from build123d import *

# Parameters (mm, degrees)
SKETCH1_W           = 14.0208
SKETCH1_H           = 7.62
BOSS_EXTRUDE1_DEPTH = 1.3081
SKETCH2_W           = 0.762
SKETCH2_H           = 0.762
CUT_EXTRUDE1_DEPTH  = 6.35
CHAMFER1_SIZE       = 0.508
SKETCH3_W           = 1.778
SKETCH3_H           = 1.778
CUT_EXTRUDE2_DEPTH  = 0.254
SKETCH4_R           = 0.762
CUT_EXTRUDE3_DEPTH  = 5.08
SKETCH5_W           = 5.0038
SKETCH5_H           = 0.6604
CUT_EXTRUDE4_DEPTH  = 8.62
SKETCH6_W           = 1.524
SKETCH6_H           = 0.381
SKETCH6_H_2         = 0.762
SKETCH6_H_3         = 1.524
CUT_EXTRUDE5_DEPTH  = 0.254
SKETCH7_W           = 1.524
SKETCH7_H           = 0.254
BOSS_EXTRUDE2_DEPTH = 3.4798
SKETCH8_W           = 0.762
SKETCH8_H           = 0.762
BOSS_EXTRUDE3_DEPTH = 12.7
CHAMFER2_SIZE       = 0.254


with BuildPart() as part:
    # Sketch1 → Boss-Extrude1 (new body, symmetric)
    with BuildSketch(Plane(origin=(0, 0, 0), x_dir=(1, 0, 0), z_dir=(0, 1, 0))):
        Rectangle(SKETCH1_W, SKETCH1_H)
    extrude(amount=BOSS_EXTRUDE1_DEPTH, both=True)

    # Sketch2 → Cut-Extrude1 (cut)
    with BuildSketch(Plane(origin=(7.0104, 0, 0), x_dir=(0, 0, -1), z_dir=(1, 0, 0))):
        Rectangle(SKETCH2_W, SKETCH2_H)
        with Locations((-2.54, 0)):
            Rectangle(SKETCH2_W, SKETCH2_H)
        with Locations((2.54, 0)):
            Rectangle(SKETCH2_W, SKETCH2_H)
    extrude(amount=-CUT_EXTRUDE1_DEPTH, mode=Mode.SUBTRACT)

    # Chamfer1
    chamfer1_edges = [part.edges().sort_by_distance(p)[0] for p in [
        (7.0104, -0.381, 2.54),
        (7.0104, 0, 2.159),
        (7.0104, 0.381, 2.54),
        (7.0104, 0, 2.921),
        (7.0104, -0.381, 0),
        (7.0104, 0, -0.381),
        (7.0104, 0.381, 0),
        (7.0104, 0, 0.381),
        (7.0104, -0.381, -2.54),
        (7.0104, 0, -2.921),
        (7.0104, 0.381, -2.54),
        (7.0104, 0, -2.159),
    ]]
    chamfer(chamfer1_edges, length=CHAMFER1_SIZE)

    # Sketch3 → Cut-Extrude2 (cut)
    with BuildSketch(Plane.ZY.offset(7.0104)):
        with Locations((-2.54, 0)):
            Rectangle(SKETCH3_W, SKETCH3_H)
        Rectangle(SKETCH3_W, SKETCH3_H)
        with Locations((2.54, 0)):
            Rectangle(SKETCH3_W, SKETCH3_H)
    extrude(amount=-CUT_EXTRUDE2_DEPTH, mode=Mode.SUBTRACT)

    # Sketch4 → Cut-Extrude3 (cut)
    with BuildSketch(Plane.ZY.offset(6.7564)):
        with Locations((-2.54, 0)):
            Circle(SKETCH4_R)
        Circle(SKETCH4_R)
        with Locations((2.54, 0)):
            Circle(SKETCH4_R)
    extrude(amount=-CUT_EXTRUDE3_DEPTH, mode=Mode.SUBTRACT)

    # Sketch5 → Cut-Extrude4 (cut, through all)
    with BuildSketch(Plane.XY.offset(3.81)):
        with Locations((0.5715, 1.3081)):
            Rectangle(SKETCH5_W, SKETCH5_H)
    extrude(amount=-CUT_EXTRUDE4_DEPTH, mode=Mode.SUBTRACT)

    # Sketch6 → Cut-Extrude5 (cut)
    with BuildSketch(Plane(origin=(0, 0.9779, 0), x_dir=(1, 0, 0), z_dir=(0, 1, 0))):
        with Locations((2.3114, 3.1115)):
            Rectangle(SKETCH6_W, SKETCH6_H)
        with Locations((2.3114, 2.54)):
            Rectangle(SKETCH6_W, SKETCH6_H_2)
        with Locations((2.3114, 1.9685)):
            Rectangle(SKETCH6_W, SKETCH6_H)
        with Locations((2.3114, 0)):
            Rectangle(SKETCH6_W, SKETCH6_H_3)
        with Locations((2.3114, -2.54)):
            Rectangle(SKETCH6_W, SKETCH6_H_3)
    extrude(amount=-CUT_EXTRUDE5_DEPTH, mode=Mode.SUBTRACT)

    # Sketch7 → Boss-Extrude2 (add)
    with BuildSketch(Plane(origin=(-1.9304, 0, 0), x_dir=(0, 0, -1), z_dir=(1, 0, 0))):
        with Locations((2.54, 1.1049)):
            Rectangle(SKETCH7_W, SKETCH7_H)
        with Locations((0, 1.1049)):
            Rectangle(SKETCH7_W, SKETCH7_H)
        with Locations((-2.54, 1.1049)):
            Rectangle(SKETCH7_W, SKETCH7_H)
    extrude(amount=BOSS_EXTRUDE2_DEPTH)

    # Sketch8 → Boss-Extrude3 (add)
    with BuildSketch(Plane(origin=(0.6604, 0, 0), x_dir=(0, 0, -1), z_dir=(1, 0, 0))):
        with Locations((-2.54, 0)):
            Rectangle(SKETCH8_W, SKETCH8_H)
        Rectangle(SKETCH8_W, SKETCH8_H)
        with Locations((2.54, 0)):
            Rectangle(SKETCH8_W, SKETCH8_H)
    extrude(amount=BOSS_EXTRUDE3_DEPTH)

    # Chamfer2
    chamfer2_edges = [part.edges().sort_by_distance(p)[0] for p in [
        (13.3604, 0, 2.921),
        (13.3604, -0.381, 2.54),
        (13.3604, 0, 2.159),
        (13.3604, 0.381, 2.54),
        (13.3604, 0, 0.381),
        (13.3604, -0.381, 0),
        (13.3604, 0, -0.381),
        (13.3604, 0.381, 0),
        (13.3604, 0, -2.159),
        (13.3604, -0.381, -2.54),
        (13.3604, 0, -2.921),
        (13.3604, 0.381, -2.54),
    ]]
    chamfer(chamfer2_edges, length=CHAMFER2_SIZE)


solid = part.part
For this review, take the finished solid that the model builds, in its own axes (mm). A direction names the side the tool comes from. Round coordinates to 2 decimals unless told otherwise and drop trailing zeros. Loops run counter-clockwise (first coordinate to the right, second up) from the corner with the lowest first, then second, coordinate; pieces in that order, holes last. Notation, with made-up numbers: (24, 88) - (73, 88) arc R23 ccw to (73, 103) - close; hole circle Ø8 at (-12, 85). An arc over 180 degrees is marked (long way). One line per item, written item: value. Start each with the question number.
Item 1: Clearance check with flat-ended pins moving along their axes: pin 1 Ø0.6 at (x, z) = (9.5, 0) entering from -Y; pin 2 Ø0.8 at (x, z) = (0.5, 1.5) entering from +Y; pin 3 Ø0.8 at (x, z) = (9, 2.5) entering from +Y. State where each tip first meets the part, or that it passes through.
Item 2: Take a section at C-C (z = -1.25). Give the boundary of the cut face in (x, y), plus the area to 3 significant figures.
Item 3: Take a section at A-A (x = -5). Give the boundary of the cut face in (y, z), plus the area to 3 significant figures.
Item 4: Take a section at B-B (x = 8.25). Give the boundary of the cut face in (y, z).
Item 5: Take a section at D-D (x = -1.25). Give the boundary of the cut face in (y, z), plus the area to 3 significant figures.
Item 6: For L1, parallel to Y at x = -3.1, z = 0; L2, parallel to X at y = 1.05, z = 3; L3, parallel to X at y = 0.6, z = 1.25, list the stretches that pass through material, from the lowest coordinate up.
Item 7: The part is to be moulded in two halves that separate along Z. For faces 4 (the flat face through (0, 0, 3.81)), 5 (the flat face through (0, 1.232, -3)), 6 (the flat face through (1, 0.978, -1)), say which applies: +Z half, -Z half, draft (parallel to the pull), parting line (faces both ways), or undercut.
Item 8: For faces 1 (the flat face through (-1.676, 0, -3)), 2 (the flat face through (2, 0.724, -3)), 3 (the flat face through (0, 1.232, 3)), list the 3-axis set-ups (+Z, -Z, +X, -X, +Y, -Y) from which the entire face can be reached by the end or side of a thin tool; tool diameter is ignored.
Answer below:
1. pin 1: stops at y = -0.38
1. pin 2: stops at y = 1.23
1. pin 3: stops at y = 0.38
2. outline: (-7.01, -1.31) - (7.01, -1.31) - (7.01, 1.31) - (3.07, 1.31) - (3.07, 0.98) - (-1.93, 0.98) - (-1.93, 1.31) - (-7.01, 1.31) - close
2. area: 35.0 mm2
3. outline: (-1.31, -3.81) - (1.31, -3.81) - (1.31, 3.81) - (-1.31, 3.81) - close; hole circle Ø1.52 at (0, -2.54); hole circle Ø1.52 at (0, 0); hole circle Ø1.52 at (0, 2.54)
3. area: 14.5 mm2
4. outline: (-0.38, -2.92) - (0.38, -2.92) - (0.38, -2.16) - (-0.38, -2.16) - close; (-0.38, -0.38) - (0.38, -0.38) - (0.38, 0.38) - (-0.38, 0.38) - close; (-0.38, 2.16) - (0.38, 2.16) - (0.38, 2.92) - (-0.38, 2.92) - close
5. outline: (-1.31, -3.81) - (0.98, -3.81) - (0.98, -3.3) - (1.23, -3.3) - (1.23, -1.78) - (0.98, -1.78) - (0.98, -0.76) - (1.23, -0.76) - (1.23, 0.76) - (0.98, 0.76) - (0.98, 1.78) - (1.23, 1.78) - (1.23, 3.3) - (0.98, 3.3) - (0.98, 3.81) - (-1.31, 3.81) - close
5. area: 18.6 mm2
6. L1: y = -1.31 to -0.76, 0.76 to 1.31
6. L2: x = -7.01 to 1.55, 3.07 to 7.01
6. L3: x = -7.01 to 7.01
7. face 4: +Z half
7. face 5: draft
7. face 6: undercut
8. face 1: -X
8. face 2: +Y
8. face 3: +Z, -Z, +Y
